Source: CAD feature listing. Evaluate the final solid. Frame: model axes, mm. A direction names the side the tool comes from. Coordinates: 2 decimals unless noted, no trailing zeros. Loops run counter-clockwise (first coordinate to the right, second up) from the corner with the lowest first, then second, coordinate; pieces in that order, holes last.
```python
from build123d import *

# Parameters (mm, degrees)
F0_R      = 4.7625
F1_DEPTH  = 1.5875
F2_R      = 3.96875
F3_DEPTH  = 8.89
F4_W      = 9.525
F4_H      = 9.525
F5_DEPTH  = 19.05
F6_SIZE   = 0.79375
F7_R      = 4.7625
F7_R_2    = 2.38125
F8_DEPTH  = 7.9375
F9_R      = 1.7272
F10_DEPTH = 9.525
F11_R     = 1.7272
F12_DEPTH = 4.1232527964


with BuildPart() as f1:
    # F0 (on Top) → F1 (new body)
    with BuildSketch(Plane.XY):
        Circle(F0_R)
    extrude(amount=F1_DEPTH)

    # F2 (on face) → F3 (join)
    with BuildSketch(Plane.XY.offset(1.5875)):
        Circle(F2_R)
    extrude(amount=F3_DEPTH)

    # F4 (on face) → F5 (join)
    with BuildSketch(Plane(origin=(0, 0, 0), x_dir=(1, 0, 0), z_dir=(0, 0, -1))):
        Rectangle(F4_W, F4_H)
    extrude(amount=F5_DEPTH)

    # F6
    f6_edges = [f1.edges().sort_by_distance(p)[0] for p in [
        (-3.96875, 0, 10.4775),
    ]]
    chamfer(f6_edges, length=F6_SIZE)

    # F7 (on face) → F8 (join)
    with BuildSketch(Plane(origin=(0, 0, -19.05), x_dir=(1, 0, 0), z_dir=(0, 0, -1))):
        Circle(F7_R)
        Circle(F7_R_2, mode=Mode.SUBTRACT)
    extrude(amount=F8_DEPTH)

    # F9 (on face) → F10 (cut, through all)
    with BuildSketch(Plane(origin=(0, 4.7625, 0), x_dir=(-1, 0, 0), z_dir=(0, 1, 0))):
        with Locations((0, -4.7625)):
            Circle(F9_R)
        with Locations((0, -14.2875)):
            Circle(F9_R)
    extrude(amount=-F10_DEPTH, mode=Mode.SUBTRACT)

    # F11 (on face) → F12 (cut, up to face)
    with BuildSketch(Plane(origin=(0, 4.7625, 0), x_dir=(-1, 0, 0), z_dir=(0, 1, 0))):
        with Locations((0, -23.01875)):
            Circle(F11_R)
    extrude(amount=-F12_DEPTH, mode=Mode.SUBTRACT)


solid = f1.part
```
Q1. Section query A-A on z = -15. Return the cut outline in (x, y).
Q2. Draft query along X for faces 5 (the flat face through (4.762, 0, -9)), 6 (the flat face through (0, 0, -19.05)), 7 (the flat face through (0, 4.762, -9)). Return one class per face: released by +X, released by -X, zero draft, split by the parting line, or undercut.
Q3. First-contact query: pin 1 Ø1.4 at (x, y) = (2.5, -3) entering from +Z; pin 2 Ø1.4 at (x, y) = (0, 0) entering from -Z; pin 3 Ø3 at (x, z) = (0, -23.02) entering from +Y. Flat tips, straight axial feed; report the tip coordinate or a pass-through.
Q4. Reachability of faces 1 (the cylindrical face through (-3.78, -2.9, 0.78)), 2 (the flat face through (-4, 4, 0)), 3 (the flat face through (-4, 4, -19.05)), 4 (the cylindrical face through (-0.62, -4.72, -22.96)) from +Z, -Z, +X, -X, +Y, -Y: full face, straight path, thin tool, end or side. Return the list, or none.
Q5. Section query D-D on z = 2.5. Return the cut outline in (x, y), then the cut area to 3 significant figures.
Q6. Section query B-B on z = -4. Return the cut outline in (x, y), then the cut area to 3 significant figures.
Q7. Section query C-C on x = -1.25. Count the separate pieces of the cut face and the enclosed holes in it, then the cut area to 3 significant figures.
Q8. Material intervals for line 1 along Z through (x, y) = (0, 0.5); line 2 along Z through (x, y) = (0, -2.5); line 3 along Z through (x, y) = (0, 2.85), sorted ascending.
Resolved:
1. outline: (-4.76, -4.76) - (-1.57, -4.76) - (-1.57, 4.76) - (-4.76, 4.76) - close; (1.57, -4.76) - (4.76, -4.76) - (4.76, 4.76) - (1.57, 4.76) - close
2. face 5: released by +X
2. face 6: undercut
2. face 7: zero draft
3. pin 1: stops at z = 10.45
3. pin 2: stops at z = -19.05
3. pin 3: stops at y = -1.85
4. face 1: +Z
4. face 2: +Z, -X, +Y
4. face 3: -Z, -X, +Y
4. face 4: -Z
5. outline: circle Ø7.94 at (0, 0)
5. area: 49.5 mm2
6. outline: (-4.76, -4.76) - (-1.55, -4.76) - (-1.55, 4.76) - (-4.76, 4.76) - close; (1.55, -4.76) - (4.76, -4.76) - (4.76, 4.76) - (1.55, 4.76) - close
6. area: 61.2 mm2
7. separate pieces: 4
7. enclosed holes: 0
7. area: 252 mm2
8. line 1: z = -19.05 to -16.01, -12.56 to -6.49, -3.04 to 10.48
8. line 2: z = -26.99 to -16.01, -12.56 to -6.49, -3.04 to 10.48
8. line 3: z = -26.99 to -24.75, -21.29 to -16.01, -12.56 to -6.49, -3.04 to 10.48
